Part model, mm, in its own coordinate system. A direction names the side the tool comes from. Coordinates: 2 decimals unless noted, no trailing zeros. Write item = value, one per line.
from build123d import *

# Parameters (mm, degrees)
BOSS_EXTRUDE1_DEPTH = 300


with BuildPart() as part:
    # Sketch1 → Boss-Extrude1 (new, symmetric)
    with BuildSketch(Plane.XY):
        with BuildLine():
            Line((-19.5072, 22.5044), (-5.7912, 22.5044))
            Line((-5.7912, 22.5044), (-5.7912, 21.0058))
            Line((-5.7912, 21.0058), (-5.0038, 21.0058))
            Line((-5.0038, 21.0058), (-5.0038, 16.51))
            Line((-5.0038, 16.51), (-10.0457, 16.51))
            Line((-10.0457, 16.51), (-10.0457, 11.680106614))
            Line((-10.0457, 11.680106614), (-4.781026704, 6.415433318))
            ThreePointArc((-4.781026704, 6.415433318), (0, 8.001), (4.781026704, 6.415433318))
            Line((4.781026704, 6.415433318), (10.0457, 11.680106614))
            Line((10.0457, 11.680106614), (10.0457, 16.51))
            Line((10.0457, 16.51), (5.0038, 16.51))
            Line((5.0038, 16.51), (5.0038, 21.0058))
            Line((5.0038, 21.0058), (5.7912, 21.0058))
            Line((5.7912, 21.0058), (5.7912, 22.5044))
            Line((5.7912, 22.5044), (19.5072, 22.5044))
            ThreePointArc((19.5072, 22.5044), (21.626540445, 21.626540445), (22.5044, 19.5072))
            Line((22.5044, 19.5072), (22.5044, 5.7912))
            Line((22.5044, 5.7912), (21.0058, 5.7912))
            Line((21.0058, 5.7912), (21.0058, 5.0038))
            Line((21.0058, 5.0038), (16.51, 5.0038))
            Line((16.51, 5.0038), (16.51, 10.0457))
            Line((16.51, 10.0457), (11.680106614, 10.0457))
            Line((11.680106614, 10.0457), (6.415433318, 4.781026704))
            ThreePointArc((6.415433318, 4.781026704), (8.001, 0), (6.415433318, -4.781026704))
            Line((6.415433318, -4.781026704), (11.680106614, -10.0457))
            Line((11.680106614, -10.0457), (16.51, -10.0457))
            Line((16.51, -10.0457), (16.51, -5.0038))
            Line((16.51, -5.0038), (21.0058, -5.0038))
            Line((21.0058, -5.0038), (21.0058, -5.7912))
            Line((21.0058, -5.7912), (22.5044, -5.7912))
            Line((22.5044, -5.7912), (22.5044, -19.5072))
            ThreePointArc((22.5044, -19.5072), (21.626540445, -21.626540445), (19.5072, -22.5044))
            Line((19.5072, -22.5044), (5.7912, -22.5044))
            Line((5.7912, -22.5044), (5.7912, -21.0058))
            Line((5.7912, -21.0058), (5.0038, -21.0058))
            Line((5.0038, -21.0058), (5.0038, -16.51))
            Line((5.0038, -16.51), (10.0457, -16.51))
            Line((10.0457, -16.51), (10.0457, -11.680106614))
            Line((10.0457, -11.680106614), (4.781026704, -6.415433318))
            ThreePointArc((4.781026704, -6.415433318), (0, -8.001), (-4.781026704, -6.415433318))
            Line((-4.781026704, -6.415433318), (-10.0457, -11.680106614))
            Line((-10.0457, -11.680106614), (-10.0457, -16.51))
            Line((-10.0457, -16.51), (-5.0038, -16.51))
            Line((-5.0038, -16.51), (-5.0038, -21.0058))
            Line((-5.0038, -21.0058), (-5.7912, -21.0058))
            Line((-5.7912, -21.0058), (-5.7912, -22.5044))
            Line((-5.7912, -22.5044), (-19.5072, -22.5044))
            ThreePointArc((-19.5072, -22.5044), (-21.626540445, -21.626540445), (-22.5044, -19.5072))
            Line((-22.5044, -19.5072), (-22.5044, -5.7912))
            Line((-22.5044, -5.7912), (-21.0058, -5.7912))
            Line((-21.0058, -5.7912), (-21.0058, -5.0038))
            Line((-21.0058, -5.0038), (-16.51, -5.0038))
            Line((-16.51, -5.0038), (-16.51, -10.0457))
            Line((-16.51, -10.0457), (-11.680106614, -10.0457))
            Line((-11.680106614, -10.0457), (-6.415433318, -4.781026704))
            ThreePointArc((-6.415433318, -4.781026704), (-8.001, 0), (-6.415433318, 4.781026704))
            Line((-6.415433318, 4.781026704), (-11.680106614, 10.0457))
            Line((-11.680106614, 10.0457), (-16.51, 10.0457))
            Line((-16.51, 10.0457), (-16.51, 5.0038))
            Line((-16.51, 5.0038), (-21.0058, 5.0038))
            Line((-21.0058, 5.0038), (-21.0058, 5.7912))
            Line((-21.0058, 5.7912), (-22.5044, 5.7912))
            Line((-22.5044, 5.7912), (-22.5044, 19.5072))
            ThreePointArc((-22.5044, 19.5072), (-21.626540445, 21.626540445), (-19.5072, 22.5044))
        make_face()
        with BuildLine():
            Line((-18.0086, 11.5443), (-13.0429, 11.5443))
            ThreePointArc((-13.0429, 11.5443), (-11.983229778, 11.983229778), (-11.5443, 13.0429))
            Line((-11.5443, 13.0429), (-11.5443, 18.0086))
            Line((-11.5443, 18.0086), (-8.7884, 18.0086))
            ThreePointArc((-8.7884, 18.0086), (-7.2898, 19.5072), (-8.7884, 21.0058))
            Line((-8.7884, 21.0058), (-19.5072, 21.0058))
            ThreePointArc((-19.5072, 21.0058), (-20.566870222, 20.566870222), (-21.0058, 19.5072))
            Line((-21.0058, 19.5072), (-21.0058, 8.7884))
            ThreePointArc((-21.0058, 8.7884), (-19.5072, 7.2898), (-18.0086, 8.7884))
            Line((-18.0086, 8.7884), (-18.0086, 11.5443))
        make_face(mode=Mode.SUBTRACT)
        with BuildLine():
            Line((1.189270603, 5.978867069), (0.976192953, 4.907653386))
            ThreePointArc((0.976192953, 4.907653386), (0, 5.0038), (-0.976192953, 4.907653386))
            Line((-0.976192953, 4.907653386), (-1.189270603, 5.978867069))
            ThreePointArc((-1.189270603, 5.978867069), (-2.332838204, 5.63196963), (-3.38675614, 5.068638757))
            Line((-3.38675614, 5.068638757), (-2.779962332, 4.160507646))
            ThreePointArc((-2.779962332, 4.160507646), (-3.538220912, 3.538220912), (-4.160507646, 2.779962332))
            Line((-4.160507646, 2.779962332), (-5.068638757, 3.38675614))
            ThreePointArc((-5.068638757, 3.38675614), (-5.63196963, 2.332838204), (-5.978867069, 1.189270603))
            Line((-5.978867069, 1.189270603), (-4.907653386, 0.976192953))
            ThreePointArc((-4.907653386, 0.976192953), (-5.0038, 0), (-4.907653386, -0.976192953))
            Line((-4.907653386, -0.976192953), (-5.978867069, -1.189270603))
            ThreePointArc((-5.978867069, -1.189270603), (-5.63196963, -2.332838204), (-5.068638757, -3.38675614))
            Line((-5.068638757, -3.38675614), (-4.160507646, -2.779962332))
            ThreePointArc((-4.160507646, -2.779962332), (-3.538220912, -3.538220912), (-2.779962332, -4.160507646))
            Line((-2.779962332, -4.160507646), (-3.38675614, -5.068638757))
            ThreePointArc((-3.38675614, -5.068638757), (-2.332838204, -5.63196963), (-1.189270603, -5.978867069))
            Line((-1.189270603, -5.978867069), (-0.976192953, -4.907653386))
            ThreePointArc((-0.976192953, -4.907653386), (0, -5.0038), (0.976192953, -4.907653386))
            Line((0.976192953, -4.907653386), (1.189270603, -5.978867069))
            ThreePointArc((1.189270603, -5.978867069), (2.332838204, -5.63196963), (3.38675614, -5.068638757))
            Line((3.38675614, -5.068638757), (2.779962332, -4.160507646))
            ThreePointArc((2.779962332, -4.160507646), (3.538220912, -3.538220912), (4.160507646, -2.779962332))
            Line((4.160507646, -2.779962332), (5.068638757, -3.38675614))
            ThreePointArc((5.068638757, -3.38675614), (5.63196963, -2.332838204), (5.978867069, -1.189270603))
            Line((5.978867069, -1.189270603), (4.907653386, -0.976192953))
            ThreePointArc((4.907653386, -0.976192953), (5.0038, 0), (4.907653386, 0.976192953))
            Line((4.907653386, 0.976192953), (5.978867069, 1.189270603))
            ThreePointArc((5.978867069, 1.189270603), (5.63196963, 2.332838204), (5.068638757, 3.38675614))
            Line((5.068638757, 3.38675614), (4.160507646, 2.779962332))
            ThreePointArc((4.160507646, 2.779962332), (3.538220912, 3.538220912), (2.779962332, 4.160507646))
            Line((2.779962332, 4.160507646), (3.38675614, 5.068638757))
            ThreePointArc((3.38675614, 5.068638757), (2.332838204, 5.63196963), (1.189270603, 5.978867069))
        make_face(mode=Mode.SUBTRACT)
        with BuildLine():
            Line((11.5443, 18.0086), (8.7884, 18.0086))
            ThreePointArc((8.7884, 18.0086), (7.2898, 19.5072), (8.7884, 21.0058))
            Line((8.7884, 21.0058), (19.5072, 21.0058))
            ThreePointArc((19.5072, 21.0058), (20.566870222, 20.566870222), (21.0058, 19.5072))
            Line((21.0058, 19.5072), (21.0058, 8.7884))
            ThreePointArc((21.0058, 8.7884), (19.5072, 7.2898), (18.0086, 8.7884))
            Line((18.0086, 8.7884), (18.0086, 11.5443))
            Line((18.0086, 11.5443), (13.0429, 11.5443))
            ThreePointArc((13.0429, 11.5443), (11.983229778, 11.983229778), (11.5443, 13.0429))
            Line((11.5443, 13.0429), (11.5443, 18.0086))
        make_face(mode=Mode.SUBTRACT)
        with BuildLine():
            Line((18.0086, -11.5443), (13.0429, -11.5443))
            ThreePointArc((13.0429, -11.5443), (11.983229778, -11.983229778), (11.5443, -13.0429))
            Line((11.5443, -13.0429), (11.5443, -18.0086))
            Line((11.5443, -18.0086), (8.7884, -18.0086))
            ThreePointArc((8.7884, -18.0086), (7.2898, -19.5072), (8.7884, -21.0058))
            Line((8.7884, -21.0058), (19.5072, -21.0058))
            ThreePointArc((19.5072, -21.0058), (20.566870222, -20.566870222), (21.0058, -19.5072))
            Line((21.0058, -19.5072), (21.0058, -8.7884))
            ThreePointArc((21.0058, -8.7884), (19.5072, -7.2898), (18.0086, -8.7884))
            Line((18.0086, -8.7884), (18.0086, -11.5443))
        make_face(mode=Mode.SUBTRACT)
        with BuildLine():
            Line((-11.5443, -18.0086), (-8.7884, -18.0086))
            ThreePointArc((-8.7884, -18.0086), (-7.2898, -19.5072), (-8.7884, -21.0058))
            Line((-8.7884, -21.0058), (-19.5072, -21.0058))
            ThreePointArc((-19.5072, -21.0058), (-20.566870222, -20.566870222), (-21.0058, -19.5072))
            Line((-21.0058, -19.5072), (-21.0058, -8.7884))
            ThreePointArc((-21.0058, -8.7884), (-19.5072, -7.2898), (-18.0086, -8.7884))
            Line((-18.0086, -8.7884), (-18.0086, -11.5443))
            Line((-18.0086, -11.5443), (-13.0429, -11.5443))
            ThreePointArc((-13.0429, -11.5443), (-11.983229778, -11.983229778), (-11.5443, -13.0429))
            Line((-11.5443, -13.0429), (-11.5443, -18.0086))
        make_face(mode=Mode.SUBTRACT)
    extrude(amount=BOSS_EXTRUDE1_DEPTH, both=True)


solid = part.part
Q1. Probe line 1 (X direction, y = 16, z = -68.5); line 2 (Y direction, x = -17, z = 67.5). List the from-to ranges inside material, lowest first. Write a range as from..to.
Model answer:
line_1 = -22.5..-21.01, -11.54..-10.05, 10.05..11.54, 21.01..22.5
line_2 = -22.5..-21.01, -11.54..-5, 5..11.54, 21.01..22.5
Q2. Saw through at A-A on z = -22. Count the separate pieces of the cut face and the enclosed holes in it, and give its area (3 significant figures).
Model answer:
separate_pieces = 1
enclosed_holes = 5
area = 563 mm²
Q3. Which spindle directions (+Z, -Z, +X, -X, +Y, -Y) get a long thin tool onto all of the face, cutting with end or side? Do faces 1 (the face through (7, 2, 300)), 2 (the face through (14, -21.006, 4)). Say none if no direction does.
Model answer:
face_1 = +Z, +X, -X, +Y, -Y
face_2 = +Z, -Z
Q4. Pin check, flat tips, straight feed: pin 1 (4 mm diameter, centred on y = 1, z = 192, fed in from +X); pin 2 (1.6 mm diameter, centred on x = 22, z = -133.5, fed in from +Y); pin 3 (1 mm diameter, centred on y = -0.5, z = 33.5, fed in from -X). Stop position of each tip, or through.
Model answer:
pin_1 = 8
pin_2 = 21.98
pin_3 = -8
